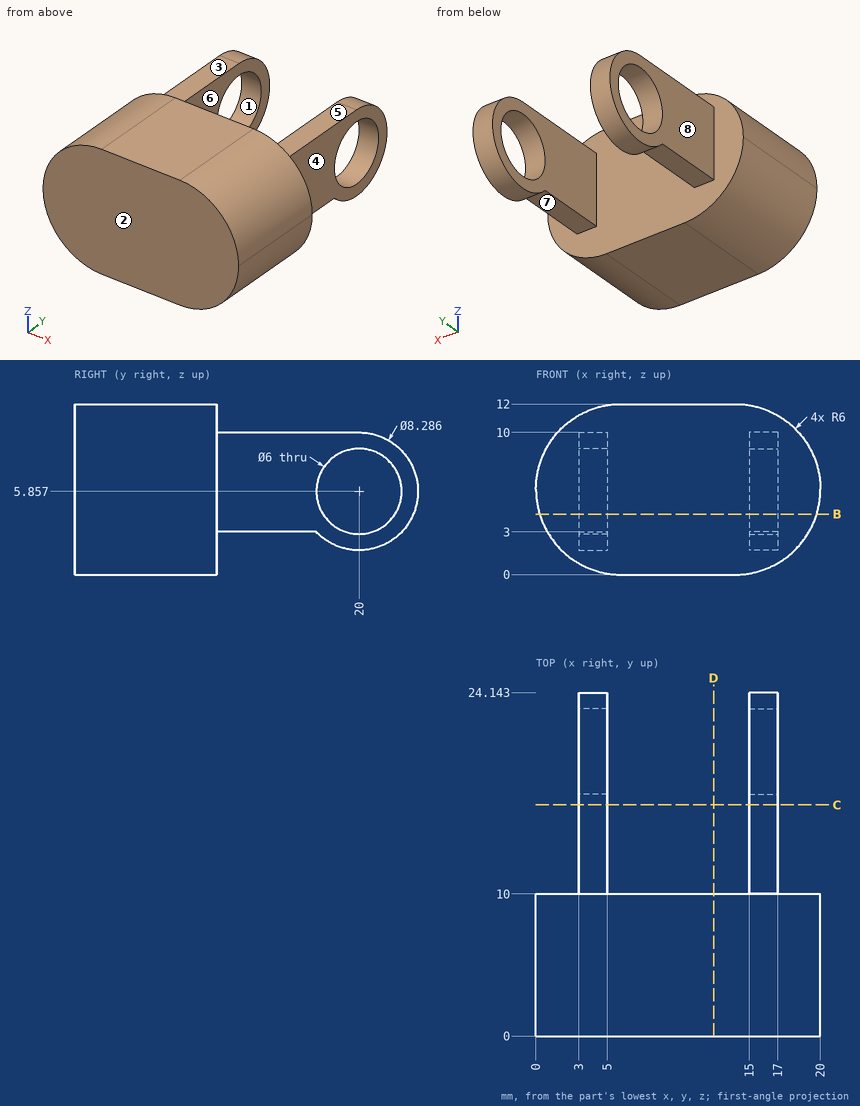
Here's the drawing with two shaded views (mm, measured from the low corner). I have some questions. A direction names the side the tool comes from. Give positions to 0.01 mm unless a question says otherwise; leave off trailing zeros. Loops run counter-clockwise (first coordinate to the right, second up) from the corner with the lowest first, then second, coordinate; pieces in that order, holes last. Notation, with made-up numbers: M -19,79.5 L 18,79.5 A24 cw 18,110.5 Z; hole C 43.25,85 d9. An arc over 180 degrees is marked long. Use one line per item in the form item = value. Start each with the question number.
Q1. If we section it at C-C (y = 16.25): Write out the boundary of the cut face in (x, z), then the cut area to 3 significant figures.
Q2. Which directions (+Z, -Z, +X, -X, +Y, -Y) give clear straight access to the entire face, cutting with the end or side of a thin tool? Please do the marked faces 4, 5, 6, 7 and 8.
Q3. Will these pins go through, and if not, where does the flat tip stop? pin 1 Ø3 at (y, z) = (18.5, 4.5) entering from -X; pin 2 Ø1 at (x, y) = (4, 13.5) entering from -Z; pin 3 Ø2.5 at (y, z) = (18, 6) entering from +X; pin 4 Ø1 at (x, y) = (13, 14.5) entering from +Z.
Q4. Thinking about a two-plate mould opening in Y: for the marked faces 1, 2 and 3, which applies, +Y half, -Y half, draft (parallel to the pull), parting line (faces both ways), or undercut?
Q5. If we section it at D-D (x = 12.5): Write out the boundary of the cut face in (y, z).
Q6. I need wall thicknesses on line 1 along X through (y, z) = (20.5, 9.75); line 2 along Y through (x, z) = (7, 2.5); line 3 along Y through (x, z) = (15.5, 5.75). Which ranges of each line are inside material? Lowest first, please.
Q7. If we section it at B-B (z = 4.25): Write out the boundary of the cut face in (x, y).
Taken from the geometry:
q1.outline = M 3,3 L 5,3 L 5,10 L 3,10 Z; M 15,3 L 17,3 L 17,10 L 15,10 Z
q1.area = 28.0 mm^2
q2.face_4 = +Z, -Z, +X, +Y
q2.face_5 = +Z, +X, -X, +Y
q2.face_6 = +Z, -Z, +Y
q2.face_7 = -Z, +X, -X
q2.face_8 = +Z, -Z, -X, +Y
q3.pin_1 = 3
q3.pin_2 = 3
q3.pin_3 = 17
q3.pin_4 = through
q4.face_1 = undercut
q4.face_2 = -Y half
q4.face_3 = draft
q5.outline = M 0,0 L 10,0 L 10,12 L 0,12 Z
q6.line_1 = 3 to 5, 15 to 17
q6.line_2 = 0 to 10
q6.line_3 = 0 to 17, 23 to 24.14
q7.outline = M 0.26,0 L 19.74,0 L 19.74,10 L 17,10 L 17,17.47 L 15,17.47 L 15,10 L 5,10 L 5,17.47 L 3,17.47 L 3,10 L 0.26,10 Z; M 3,22.53 L 5,22.53 L 5,23.82 L 3,23.82 Z; M 15,22.53 L 17,22.53 L 17,23.82 L 15,23.82 Z
